Geometry check sheet. Reference: the model listing, model coordinates, mm. A direction names the side the tool comes from. Give positions to 0.01 mm unless a question says otherwise; leave off trailing zeros. Loops run counter-clockwise (first coordinate to the right, second up) from the corner with the lowest first, then second, coordinate; pieces in that order, holes last. Notation, with made-up numbers: (-38, -13.75) -> (-20, -13.75) arc R24 ccw to (-20, 25.25) -> close; hole circle Ø7 at (15.25, 41). An arc over 180 degrees is marked (long way). One line per item, written item: value. Start each with the question number.
(1) Gauge pin test, flat ends, axial feed: pin 1 Ø1.5 at (x, z) = (-12, 1.5) entering from +Y; pin 2 Ø1 at (x, z) = (4.5, 5) entering from +Y; pin 3 Ø1 at (x, z) = (-7, 1) entering from +Y. Record the tip position at first contact, or that the pin passes through.
(2) Scan lines: line 1 along Y through (x, z) = (-4.5, 6.25); line 2 along Y through (x, z) = (-1, 3); line 3 along X through (y, z) = (13, 2.5). Record each from-to range of solid material in increasing order. Write a range as from..to.
(3) Sectioned sample at A-A, the plane y = 16. Record the cut outline in (x, z), then the cut area to 3 significant figures.
(4) Tool access check on faces 4 (the face through (4.83, 15.75, 3.13)), 5 (the face through (-9.011, -15.382, 3.131)). Record the directions out of +Z, -Z, +X, -X, +Y, -Y that give a thin tool (end or side, any length) a straight path to the whole face; none if there is none.
(5) Draft check along X on faces 1 (the face through (-1.5, 3.58, 3.13)), 2 (the face through (-9.551, 18.426, 3.131)), 3 (the face through (-9, 6, 0)). Enter one of: pulls with the +X half, pulls with the -X half, needs draft (parallel to the pull), parting line crosses it, or undercut.
(6) Sectioned sample at D-D, the plane x = -16. Record the cut outline in (y, z), then the cut area to 3 significant figures.
(7) Sectioned sample at C-C, the plane z = 1. Record the cut outline in (x, y), then the cut area to 3 significant figures.
(8) Sectioned sample at B-B, the plane x = -3.5. Record the cut outline in (y, z), then the cut area to 3 significant figures.
from build123d import *

# Parameters (mm, degrees)
F1_DEPTH = 6.35


with BuildPart() as f1:
    # F0 (on Top) → F1 (new body)
    with BuildSketch(Plane.XY):
        with BuildLine():
            ThreePointArc((-18.731252, -17.982043), (-8.866157, -15.404018), (-0.284833, -20.911031))
            ThreePointArc((-0.284833, -20.911031), (2.246411, -22.009452), (4.285943, -20.150948))
            Line((4.285943, -20.150948), (7.392956, -8.357487))
            ThreePointArc((7.392956, -8.357487), (7.28039, -4.743075), (5.212962, -1.776192))
            Line((5.212962, -1.776192), (-8.396228, 9.082717))
            ThreePointArc((-8.396228, 9.082717), (-9.459502, 18.542219), (0, 19.605493))
            Line((0, 19.605493), (9.795078, 11.789902))
            ThreePointArc((9.795078, 11.789902), (12.481031, 11.486723), (13.919272, 13.775331))
            Line((13.919272, 13.775331), (13.919272, 14.344105))
            ThreePointArc((13.919272, 14.344105), (-4.198114, 32.46149), (-22.315499, 14.344105))
            Line((-22.315499, 14.344105), (-22.845562, -15.94463))
            ThreePointArc((-22.845562, -15.94463), (-21.433128, -18.265271), (-18.731252, -17.982043))
        make_face()
    extrude(amount=F1_DEPTH)


solid = f1.part
Calculated:
1. pin 1: stops at y = 31.03
1. pin 2: stops at y = 30.5
1. pin 3: stops at y = 32.31
2. line 1: y = -16.95..5.97, 21.07..32.46
2. line 2: y = -19.94..3.18, 20.27..32.18
2. line 3: x = -22.34..-10.79, 8.28..13.8
3. outline: (-22.24, 0) -> (-10.72, 0) -> (-10.72, 6.35) -> (-22.24, 6.35) -> close; (4.52, 0) -> (13.84, 0) -> (13.84, 6.35) -> (4.52, 6.35) -> close
3. area: 132 mm2
4. face 4: +Z, -Z
4. face 5: +Z, -Z, -Y
5. face 1: pulls with the +X half
5. face 2: undercut
5. face 3: needs draft
6. outline: (-16.33, 0) -> (28.09, 0) -> (28.09, 6.35) -> (-16.33, 6.35) -> close
6. area: 282 mm2
7. outline: (-22.85, -15.94) arc R2.54 ccw to (-18.73, -17.98) arc R12.7 cw to (-0.28, -20.91) arc R2.54 ccw to (4.29, -20.15) -> (7.39, -8.36) arc R6.35 ccw to (5.21, -1.78) -> (-8.4, 9.08) arc R6.73 cw to (0, 19.61) -> (9.8, 11.79) arc R2.54 ccw to (13.92, 13.78) -> (13.92, 14.34) arc R18.12 ccw to (-22.32, 14.34) -> close
7. area: 1,210 mm2
8. outline: (-17.6, 0) -> (5.18, 0) -> (5.18, 6.35) -> (-17.6, 6.35) -> close; (21.04, 0) -> (32.45, 0) -> (32.45, 6.35) -> (21.04, 6.35) -> close
8. area: 217 mm2
